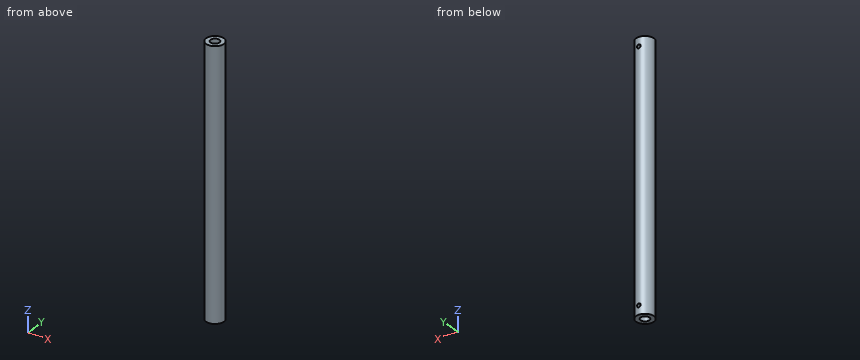
```python
from build123d import *

# Parameters (mm, degrees)
SKETCH1_R                = 15
SKETCH1_R_2              = 7.5
BOSS_EXTRUDE1_DEPTH      = 221.25
BOSS_EXTRUDE1_DEPTH_BACK = 221.25
SKETCH3_R                = 3.1
CUT_EXTRUDE1_DEPTH       = 16


with BuildPart() as part:
    # Sketch1 → Boss-Extrude1 (new body, two sides)
    with BuildSketch(Plane.XY) as boss_extrude1_sk:
        Circle(SKETCH1_R)
        Circle(SKETCH1_R_2, mode=Mode.SUBTRACT)
    extrude(amount=BOSS_EXTRUDE1_DEPTH)
    extrude(boss_extrude1_sk.sketch, amount=-BOSS_EXTRUDE1_DEPTH_BACK)

    # Sketch3 → Cut-Extrude1 (cut, through all)
    with BuildSketch(Plane(origin=(0, 0, 0), x_dir=(1, 0, 0), z_dir=(0, 1, 0))):
        with Locations((0, 206.25)):
            Circle(SKETCH3_R)
    cut_extrude1 = extrude(amount=CUT_EXTRUDE1_DEPTH, mode=Mode.SUBTRACT)

    # Mirror1: Cut-Extrude1 across plane
    add(cut_extrude1.mirror(Plane.XY), mode=Mode.SUBTRACT)


solid = part.part
```
Geometry check sheet. Reference: the model listing, model coordinates, mm. Give positions to 0.01 mm unless a question says otherwise; leave off trailing zeros. Order: outer loops, then holes, each group sorted by start corner. A loop starts at its lowest first (then second) coordinate and runs counter-clockwise, first axis right, second up.
1. Gauge pin test, flat ends, axial feed: pin 1 Ø12 at (x, y) = (0, 0) entering from -Z; pin 2 Ø6 at (x, z) = (6.5, -145.5) entering from +Y. Record the tip position at first contact, or that the pin passes through.
2. Thickness scan on L1, parallel to Z at x = 0, y = 10; L2, parallel to Y at x = 0, z = 139; L3, parallel to X at y = 13, z = 206. Record the ranges inside material, lowest first.
3. Section check A-A, the plane y = 0. Enter the section's corners in (x, z), and give its area (3 significant figures).
4. Section check B-B, the plane z = -96. Enter the section's corners in (x, y).
Values follow:
1. pin 1: passes through
1. pin 2: stops at y = 14.59
2. L1: z = -221.25 to -209.35, -203.15 to 203.15, 209.35 to 221.25
2. L2: y = -15 to -7.5, 7.5 to 15
2. L3: x = -7.48 to -3.09, 3.09 to 7.48
3. outline: (-15, -221.25) - (-7.5, -221.25) - (-7.5, 221.25) - (-15, 221.25) - close; (7.5, -221.25) - (15, -221.25) - (15, 221.25) - (7.5, 221.25) - close
3. area: 6,640 mm2
4. outline: circle Ø30 at (0, 0); hole circle Ø15 at (0, 0)
